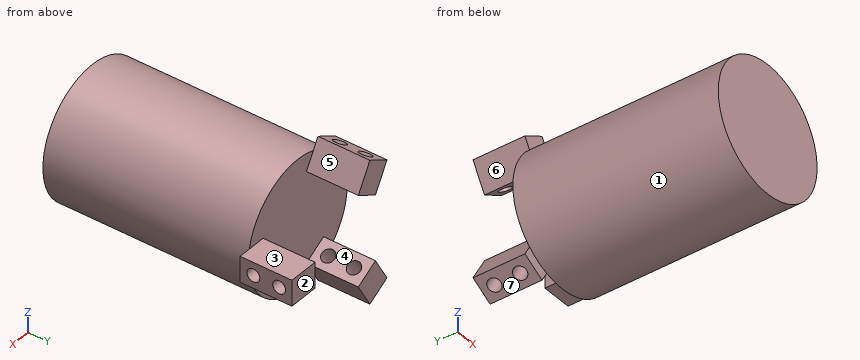
Autodesk Inventor part; units mm, degrees
ref_plane "YZ Plane" through (0, 0, 0) normal (1, 0, 0) x (0, 1, 0)
ref_plane "XZ Plane" through (0, 0, 0) normal (0, 1, 0) x (-1, 0, 0)
ref_plane "XY Plane" through (0, 0, 0) normal (0, 0, 1) x (1, 0, 0)
sketch "Sketch1" plane through (0, 0, 0) normal (0, 1, 0) x (-1, 0, 0)
  circle A0 centre (0, 0) radius 15
  dimension "d0" = 30
extrude "Extrusion1" add sketch "Sketch1" along normal blind 47.9
sketch "Sketch2" plane through (0, 47.9, 0) normal (0, 1, 0) x (1, 0, 0)
  circle A0 centre (0, 0) radius 10.5
  line L0 (10.5, 0) -> (10.5, 3)
  line L1 (10.5, 3) -> (17.5, 3)
  line L2 (17.5, 3) -> (17.5, -3)
  line L3 (17.5, -3) -> (10.5, -3)
  line L4 (10.5, -3) -> (10.5, 0)
  line L5 (-5.25, 9.0933) -> (-7.8481, 7.5933)
  line L6 (-7.8481, 7.5933) -> (-11.3481, 13.6554)
  line L7 (-11.3481, 13.6554) -> (-6.1519, 16.6554)
  line L8 (-6.1519, 16.6554) -> (-2.6519, 10.5933)
  line L9 (-2.6519, 10.5933) -> (-5.25, 9.0933)
  line L10 (-5.25, -9.0933) -> (-2.6519, -10.5933)
  line L11 (-2.6519, -10.5933) -> (-6.1519, -16.6554)
  line L12 (-6.1519, -16.6554) -> (-11.3481, -13.6554)
  line L13 (-11.3481, -13.6554) -> (-7.8481, -7.5933)
  line L14 (-7.8481, -7.5933) -> (-5.25, -9.0933)
  line L15 (0, 0) -> (-5.25, 9.0933)
  line L16 (0, 0) -> (10.5, 0)
  dimension "d4" = 21
  dimension "d5" = 3
  dimension "d6" = 7
  dimension "d7" = 6
  dimension "d10" = 360
  dimension "d12" = 120
extrude "Extrusion2" add sketch "Sketch2" along normal blind 12.1 contours L10 L11 L12 L13 L14 | L5 L6 L7 L8 L9 | L0 L1 L2 L3 L4
sketch "Sketch4" plane through (17.5, 47.9, 3) normal (1, 0, 0) x (0, 0, -1)
  line L0 (6, 12.1) -> (0, 12.1)
  line L1 (3, 12.1) -> (3, 9.1)
  line L2 (3, 9.1) -> (3, 3.1)
  circle A0 centre (3, 9.1) radius 1.5
  circle A1 centre (3, 3.1) radius 1.5
  point P0 (3, -47.9)
  dimension "d15" = 3
  dimension "d16" = 6
  dimension "d17" = 3
  dimension "d18" = 3
extrude "Extrusion3" cut sketch "Sketch4" against normal through all
sketch "Sketch5" plane through (-6.1519, 47.9, 16.6554) normal (-0.5, 0, 0.866) x (0.866, 0, 0.5)
  line L0 (-6, 12.1) -> (0, 12.1)
  line L1 (-3, 12.1) -> (-3, 9.1)
  line L2 (-3, 9.1) -> (-3, 3.1)
  circle A0 centre (-3, 9.1) radius 1.5
  circle A1 centre (-3, 3.1) radius 1.5
  point P0 (-3, -47.9)
  dimension "d21" = 3
  dimension "d22" = 6
  dimension "d23" = 3
  dimension "d24" = 3
extrude "Extrusion4" cut sketch "Sketch5" against normal through all
sketch "Sketch6" plane through (-11.3481, 47.9, -13.6554) normal (-0.5, 0, -0.866) x (-0.866, 0, 0.5)
  line L0 (8.2279, 0) -> (-14.2279, 0)
  line L1 (0, 12.1) -> (-6, 12.1)
  line L2 (-3, 12.1) -> (-3, 9.1)
  line L3 (-3, 9.1) -> (-3, 3.1)
  circle A0 centre (-3, 9.1) radius 1.5
  circle A1 centre (-3, 3.1) radius 1.5
  point P0 (-3, -47.9)
  dimension "d27" = 3
  dimension "d28" = 6
  dimension "d29" = 3
  dimension "d30" = 3
extrude "Extrusion5" cut sketch "Sketch6" against normal through all
properties part number "Cilindro" material "Aluminum 6061"
Geometry: final body of the model. Coordinates: model frame, mm. Face numbers are marked on the shaded views. A direction names the side the tool comes from. Give positions to 0.01 mm unless a question says otherwise; leave off trailing zeros. Order: outer loops, then holes, each group sorted by start corner. A loop starts at its lowest first (then second) coordinate and runs counter-clockwise, first axis right, second up. Notation, with made-up numbers: (2.25, 33.25) -> (8.25, 33.25) arc R33 ccw to (8.25, 70.25) -> close; hole circle Ø4 at (46.25, -23). An arc over 180 degrees is marked (long way). Answer as a JSON object with one key per item and string values.
Q1. Section B-B (x = 12). Output: boundary loops of the cut face in (y, z).
Entries:
{"outline": "(0, -9) -> (47.9, -9) -> (47.9, -3) -> (60, -3) -> (60, 3) -> (47.9, 3) -> (47.9, 9) -> (0, 9) -> close; hole circle Ø3 at (51, 0); hole circle Ø3 at (57, 0)"}
Q2. Draft query along Z for the marked faces 1, 2, 3 and 4. Return one class per face: released by +Z, released by -Z, zero draft, split by the parting line, or undercut.
Entries:
{"face 1": "split by the parting line", "face 2": "zero draft", "face 3": "released by +Z", "face 4": "undercut"}
Q3. First-contact query: pin 1 (1.8 mm diameter, centred on y = 51, z = 0, fed in from +X); pin 2 (3.5 mm diameter, centred on x = 13.5, y = 55.5, fed in from +Z); pin 3 (2 mm diameter, centred on y = 27.5, z = 6, fed in from +X); pin 4 (2.5 mm diameter, centred on x = -8.5, z = 14, fed in from -Y). Flat tips, straight axial feed; report the tip coordinate or a pass-through.
Entries:
{"pin 1": "passes through", "pin 2": "stops at z = 3", "pin 3": "stops at x = 14.14", "pin 4": "stops at y = 47.9"}
Q4. Material intervals for probe 1 along Y at (x, z) = (12.5, 0); probe 2 along Z at (x, y) = (14.5, 57); probe 3 along Y at (x, z) = (-2, -1), sorted ascending.
Entries:
{"probe 1": "y = 0 to 49.5, 52.5 to 55.5, 58.5 to 60", "probe 2": "z = -3 to -1.5, 1.5 to 3", "probe 3": "y = 0 to 47.9"}
Q5. Access query for the marked faces 5, 6 and 7. Directions: +Z, -Z, +X, -X, +Y, -Y. A direction counts if a zero-diameter tool reaches every point of the face in a straight line with its end or side. Return the directions, or none.
Entries:
{"face 5": "+Z, +X, +Y", "face 6": "-X, +Y", "face 7": "-Z, -X, +Y, -Y"}
Q6. Section D-D (y = 14.5). Output: boundary loops of the cut face in (x, z), plus the area to 3 significant figures.
Entries:
{"outline": "circle Ø30 at (0, 0)", "area": "707 mm^2"}
Q7. Section C-C (y = 57). Output: boundary loops of the cut face in (x, z), plus the area to 3 significant figures.
Entries:
{"outline": "(-11.35, -13.66) -> (-10.05, -14.41) -> (-6.55, -8.34) -> (-7.85, -7.59) -> close; (-11.35, 13.66) -> (-7.85, 7.59) -> (-6.55, 8.34) -> (-10.05, 14.41) -> close; (-7.45, -15.91) -> (-6.15, -16.66) -> (-2.65, -10.59) -> (-3.95, -9.84) -> close; (-7.45, 15.91) -> (-3.95, 9.84) -> (-2.65, 10.59) -> (-6.15, 16.66) -> close; (10.5, -3) -> (17.5, -3) -> (17.5, -1.5) -> (10.5, -1.5) -> close; (10.5, 1.5) -> (17.5, 1.5) -> (17.5, 3) -> (10.5, 3) -> close", "area": "63.0 mm^2"}
Q8. Section A-A (z = 0). Output: boundary loops of the cut face in (x, y).
Entries:
{"outline": "(-15, 0) -> (15, 0) -> (15, 47.9) -> (17.5, 47.9) -> (17.5, 49.5) -> (10.5, 49.5) -> (10.5, 47.9) -> (-15, 47.9) -> close; (10.5, 52.5) -> (17.5, 52.5) -> (17.5, 55.5) -> (10.5, 55.5) -> close; (10.5, 58.5) -> (17.5, 58.5) -> (17.5, 60) -> (10.5, 60) -> close"}
